Read the model definition and answer for the solid it produces. Units are mm, in the model's axes. Face numbers are marked on the shaded views. Coordinates: 2 decimals unless noted, no trailing zeros. Write each loop counter-clockwise with the first axis right and the second up, starting at its lowest first coordinate (ties: lowest second). Pieces come first, ordered by that corner, then holes.
(1) The mould has two halves that part along Y. Classify the marked faces 1 and 2: +Y half, -Y half, draft (parallel to the pull), parting line (faces both ways), or undercut.
(2) Section C-C on y = 1.7 is taken. State how many separate pieces and enclosed holes the cut face has, then the cut area to 3 significant figures.
(3) Section B-B on x = -20.5 is taken. Write down the section's boundary in (y, z), then the cut area to 3 significant figures.
(4) Section A-A on z = 6.35 is taken. Write down the section's boundary in (x, y), then the cut area to 3 significant figures.
(5) Find the intervals of material crossed by probe 1 along Z at (x, y) = (5.08, 1.2); probe 2 along X at (y, z) = (1.2, 163.83); probe 3 along Z at (x, y) = (5.5, 0.6), in increasing order.
(6) Given pin 1 (0.8 mm diameter, centred on x = -28.5, y = 1, fed in from +Z); pin 2 (8 mm diameter, centred on x = -13.5, z = 116, fed in from +Y); pin 3 (1.3 mm diameter, centred on y = 1, z = 147.5, fed in from -X); pin 4 (1.5 mm diameter, centred on y = 0.5, z = 59, fed in from -X), each flat-ended and moving along its own axis, determine where each tip first touches the part or whether it passes through.
(7) Section D-D on z = 145 is taken. Write down the section's boundary in (x, y), then the cut area to 3 significant figures.
Autodesk Inventor part; units mm, degrees
ref_plane "YZ Plane" through (0, 0, 0) normal (1, 0, 0) x (0, 1, 0)
ref_plane "XZ Plane" through (0, 0, 0) normal (0, 1, 0) x (-1, 0, 0)
ref_plane "XY Plane" through (0, 0, 0) normal (0, 0, 1) x (1, 0, 0)
sketch "Sketch1" plane through (0, 0, 0) normal (0, 1, 0) x (-1, 0, 0)
  circle A0 centre (-5.08, 6.35) radius 1.75
  circle A1 centre (-5.08, 6.35) radius 1.75
  arc A2 (-5.08, 11.43) -> (-5.08, 1.27) centre (-5.08, 6.35) ccw
  line L0 (0, 11.43) -> (0, 59.8834)
  line L1 (-5.08, 1.27) -> (5.0316, 1.27)
  line L2 (5.0316, 1.27) -> (5.0316, 63.0584)
  line L3 (-5.08, 11.43) -> (0, 11.43)
  line L4 (0, 11.43) -> (0, 59.8834)
  line L5 (5.0316, 63.0584) -> (42.3132, 63.0584)
  line L6 (5.0316, 63.0584) -> (42.3132, 63.0584)
  line L7 (44.0632, 64.8084) -> (44.0632, 105.3716)
  line L8 (44.0632, 64.8084) -> (44.0632, 105.3716)
  line L9 (42.3132, 107.1216) -> (5.0316, 107.1216)
  line L10 (42.3132, 107.1216) -> (5.0316, 107.1216)
  line L11 (5.0316, 107.1216) -> (5.0316, 168.91)
  circle A3 centre (-5.08, 163.83) radius 1.75
  circle A4 centre (-5.08, 163.83) radius 1.75
  arc A5 (-5.08, 168.91) -> (-5.08, 158.75) centre (-5.08, 163.83) ccw
  line L12 (0, 110.2966) -> (0, 158.75)
  line L13 (-5.08, 168.91) -> (5.0316, 168.91)
  line L14 (0, 59.8834) -> (0, 158.75)
  line L15 (0, 158.75) -> (-5.08, 158.75)
  arc A6 (8.0362, 72.5946) -> (9.5362, 71.0946) centre (8.0362, 71.0946) ccw
  arc A7 (8.0362, 72.5946) -> (9.5362, 71.0946) centre (8.0362, 71.0946) ccw
  arc A8 (34.527, 71.0946) -> (36.027, 72.5946) centre (36.027, 71.0946) ccw
  arc A9 (34.527, 71.0946) -> (36.027, 72.5946) centre (36.027, 71.0946) ccw
  arc A10 (36.027, 97.5854) -> (34.527, 99.0854) centre (36.027, 99.0854) ccw
  arc A11 (36.027, 97.5854) -> (34.527, 99.0854) centre (36.027, 99.0854) ccw
  arc A12 (9.5362, 99.0854) -> (8.0362, 97.5854) centre (8.0362, 99.0854) ccw
  arc A13 (9.5362, 99.0854) -> (8.0362, 97.5854) centre (8.0362, 99.0854) ccw
  arc A14 (8.0362, 68.09) -> (11.0408, 71.0946) centre (8.0362, 71.0946) ccw
  arc A15 (33.0224, 71.0946) -> (36.027, 68.09) centre (36.027, 71.0946) ccw
  line L16 (11.0408, 99.0854) -> (9.5362, 99.0854)
  line L17 (36.027, 68.09) -> (8.0362, 68.09)
  line L18 (8.0362, 68.09) -> (36.027, 68.09)
  line L19 (5.0316, 99.0854) -> (5.0316, 71.0946)
  line L20 (5.0316, 71.0946) -> (5.0316, 99.0854)
  line L21 (8.0362, 102.09) -> (36.027, 102.09)
  line L22 (8.0362, 102.09) -> (36.027, 102.09)
  line L23 (39.0316, 71.0946) -> (39.0316, 99.0854)
  line L24 (39.0316, 71.0946) -> (39.0316, 99.0854)
  line L25 (33.0224, 71.0946) -> (34.527, 71.0946)
  line L26 (34.527, 71.0946) -> (33.0224, 71.0946)
  line L27 (36.027, 72.5946) -> (36.027, 74.0992)
  line L28 (36.027, 72.5946) -> (36.027, 74.0992)
  line L29 (9.5362, 71.0946) -> (11.0408, 71.0946)
  line L30 (11.0408, 71.0946) -> (9.5362, 71.0946)
  line L31 (8.0362, 74.0992) -> (8.0362, 72.5946)
  line L32 (8.0362, 72.5946) -> (8.0362, 74.0992)
  line L33 (8.0362, 96.0808) -> (8.0362, 97.5854)
  line L34 (8.0362, 96.0808) -> (8.0362, 97.5854)
  arc A16 (11.0408, 99.0854) -> (8.0362, 102.09) centre (8.0362, 99.0854) ccw
  line L35 (9.5362, 99.0854) -> (11.0408, 99.0854)
  line L36 (36.027, 97.5854) -> (36.027, 96.0808)
  line L37 (36.027, 96.0808) -> (36.027, 97.5854)
  line L38 (33.0224, 99.0854) -> (34.527, 99.0854)
  line L39 (34.527, 99.0854) -> (33.0224, 99.0854)
  arc A17 (36.027, 96.0808) -> (39.0316, 99.0854) centre (36.027, 99.0854) ccw
  arc A18 (36.027, 102.09) -> (33.0224, 99.0854) centre (36.027, 99.0854) ccw
  arc A19 (33.0224, 71.0946) -> (36.027, 68.09) centre (36.027, 71.0946) ccw
  arc A20 (39.0316, 71.0946) -> (36.027, 74.0992) centre (36.027, 71.0946) ccw
  arc A21 (8.0362, 68.09) -> (11.0408, 71.0946) centre (8.0362, 71.0946) ccw
  arc A22 (8.0362, 74.0992) -> (5.0316, 71.0946) centre (8.0362, 71.0946) ccw
  arc A23 (11.0408, 99.0854) -> (8.0362, 102.09) centre (8.0362, 99.0854) ccw
  arc A24 (5.0316, 99.0854) -> (8.0362, 96.0808) centre (8.0362, 99.0854) ccw
  arc A25 (44.0632, 105.3716) -> (42.3132, 107.1216) centre (42.3132, 105.3716) ccw
  arc A26 (42.3132, 63.0584) -> (44.0632, 64.8084) centre (42.3132, 64.8084) ccw
  point P0 (0, 0)
  point P1 (0, 0)
  point P2 (3.175, 59.8834)
extrude "Extrusion1" add sketch "Sketch1" along normal blind 2.54
fillet "Fillet1" radius 6.35 2 edges at (0, 1.27, 11.43) (0, 1.27, 158.75)
fillet "Fillet2" radius 3.175 2 edges at (-5.0316, 1.27, 1.27) (-5.0316, 1.27, 168.91)
fillet "Fillet3" radius 19.05 2 edges at (-5.0316, 1.27, 107.1216) (-5.0316, 1.27, 63.0584)
properties part number "CameraBracket"
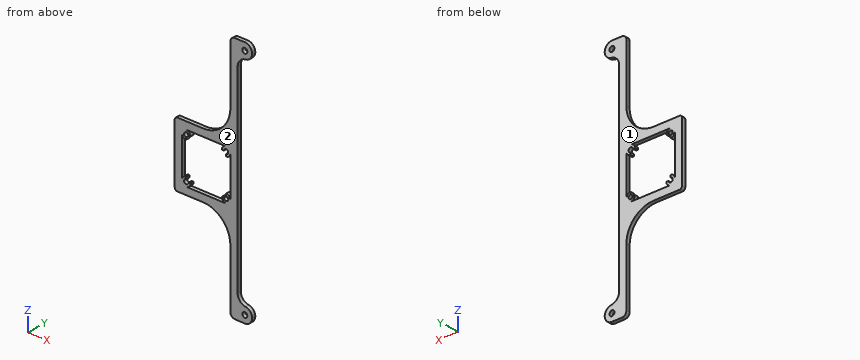
Response:
1. face 1: +Y half
1. face 2: -Y half
2. separate pieces: 1
2. enclosed holes: 3
2. area: 1,810 mm2
3. outline: (0, 62.72) - (2.54, 62.72) - (2.54, 68.09) - (0, 68.09) - close; (0, 102.09) - (2.54, 102.09) - (2.54, 107.46) - (0, 107.46) - close
3. area: 27.3 mm2
4. outline: (-5.03, 0) - (3.33, 0) - (3.33, 2.54) - (-5.03, 2.54) - close; (6.83, 0) - (10.16, 0) - (10.16, 2.54) - (6.83, 2.54) - close
4. area: 29.7 mm2
5. probe 1: z = 1.27 to 4.6, 8.1 to 11.49, 158.69 to 162.08, 165.58 to 168.91
5. probe 2: x = -5.03 to 3.33, 6.83 to 10.16
5. probe 3: z = 1.29 to 4.65, 8.05 to 11.42, 158.76 to 162.13, 165.53 to 168.89
6. pin 1: stops at z = 107.12
6. pin 2: passes through
6. pin 3: stops at x = -5.03
6. pin 4: stops at x = -13.35
7. outline: (-5.03, 0) - (0, 0) - (0, 2.54) - (-5.03, 2.54) - close
7. area: 12.8 mm2
